Model file for the job. Use its own axes, mm. Face numbers are marked on the shaded views. A direction names the side the tool comes from. Round coordinates to 2 decimals unless told otherwise and drop trailing zeros. Order: outer loops, then holes, each group sorted by start corner. A loop starts at its lowest first (then second) coordinate and runs counter-clockwise, first axis right, second up. Notation, with made-up numbers: (53, 64.5) -> (59, 64.5) arc R24 cw to (59, 90.5) -> close; hole circle Ø11 at (43.25, 20). An arc over 180 degrees is marked (long way). Put each result on its own line as item: value. Start each with the question number.
Q1. Cut at A-A, the plane x = 178.5. List the corners of the cut face in (y, z).
Q2. Cut at C-C, the plane x = 63. List the corners of the cut face in (y, z).
Q3. Probe L1, parallel to Z at x = 64, y = 28.5; L2, parallel to X at y = 44.5, z = -21.5; L3, parallel to Z at x = 27.5, y = 46. List the from-to ranges inside material, lowest first.
Q4. 3-axis set-ups, long thin cutter, end or side, ignore diameter. For the marked faces 1, 2 and 3: which of +Z, -Z, +X, -X, +Y, -Y reach the whole face in a straight line?
Q5. Cut at B-B, the plane z = -132.5. List the corners of the cut face in (x, y), and give its area (3 significant figures).
Q6. Cut at D-D, the plane z = -160. List the corners of the cut face in (x, y), and give its area (3 significant figures).
Q7. Pull direction X, two halves, no side cores. Call the marked faces 4, 5, 6 and 7: released by +X, released by -X, zero draft, split by the parting line, or undercut.
Q8. Flat gauge pins, fed straight in: P1, Ø3, axis at y = 14, z = -142.5, coming from the +X side; P2, Ø2.5, axis at x = 47.5, y = 30, coming from the +Z side; P3, Ø6, axis at x = 162, z = -55, coming from the -Y side; P4, Ø6, axis at x = 156, z = -109, coming from the -Y side. Where does each tip first touch, or does it go through?
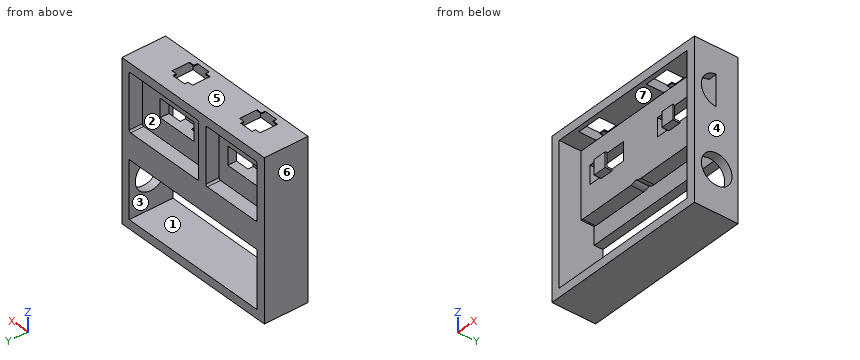
from build123d import *

# Parameters (mm, degrees)
SKETCH2_W            = 195
SKETCH2_H            = 180
BOSS_EXTRUDE1_DEPTH  = 50
CUT_EXTRUDE1_DEPTH   = 15
BOSS_EXTRUDE4_DEPTH  = 50
SKETCH14_W           = 70
SKETCH14_H           = 65
SKETCH14_W_2         = 95
BOSS_EXTRUDE8_DEPTH  = 35
SHELL2_OUTLINE_W     = 175
SHELL2_OUTLINE_H     = 65
SHELL2_DEPTH         = 75
SHELL2_2_OUTLINE_W   = 175
SHELL2_2_OUTLINE_H   = 95
SHELL2_2_DEPTH       = 25
SHELL2_START         = 25
SHELL2_3_DEPTH       = 15
SKETCH15_W           = 46
SKETCH15_H           = 21
CUT_EXTRUDE2_DEPTH   = 10
SKETCH16_W           = 46
SKETCH16_H           = 21
CUT_EXTRUDE3_DEPTH   = 10
SKETCH17_W           = 7.5
SKETCH17_H           = 8
BOSS_EXTRUDE10_DEPTH = 2
SKETCH18_W           = 15
SKETCH18_H           = 2
BOSS_EXTRUDE11_DEPTH = 15
CUT_EXTRUDE5_DEPTH   = 10
CUT_EXTRUDE6_DEPTH   = 9
SKETCH25_W           = 7.379331851
SKETCH25_H           = 8
SKETCH25_W_2         = 7.620668149
BOSS_EXTRUDE12_DEPTH = 2
SKETCH26_W           = 15
SKETCH26_H           = 2
BOSS_EXTRUDE13_DEPTH = 15
SKETCH27_R           = 17.5
CUT_EXTRUDE10_DEPTH  = 10
BOSS_EXTRUDE14_START = -10
BOSS_EXTRUDE14_DEPTH = 10


# Read off the part's stored shape, not the designer's step: Shell2
with BuildPart() as part:
    # Sketch2 → Boss-Extrude1 (new body)
    with BuildSketch(Plane(origin=(0, 0, 0), x_dir=(1, 0, 0), z_dir=(0, 1, 0))):
        with Locations((97.5, 90)):
            Rectangle(SKETCH2_W, SKETCH2_H)
    extrude(amount=BOSS_EXTRUDE1_DEPTH)

    # Sketch3 → Cut-Extrude1 (cut)
    with BuildSketch(Plane(origin=(0, 50, 0), x_dir=(1, 0, 0), z_dir=(0, 1, 0))):
        with BuildLine():
            Line((90, 12), (90, 73))
            ThreePointArc((90, 73), (90.585786438, 74.414213562), (92, 75))
            Line((92, 75), (183, 75))
            ThreePointArc((183, 75), (184.414213562, 74.414213562), (185, 73))
            Line((185, 73), (185, 12))
            ThreePointArc((185, 12), (184.414213562, 10.585786438), (183, 10))
            Line((183, 10), (92, 10))
            ThreePointArc((92, 10), (90.585786438, 10.585786438), (90, 12))
        make_face()
        with BuildLine():
            Line((12, 10), (78, 10))
            ThreePointArc((78, 10), (79.414213562, 10.585786438), (80, 12))
            Line((80, 12), (80, 73))
            ThreePointArc((80, 73), (79.414213562, 74.414213562), (78, 75))
            Line((78, 75), (12, 75))
            ThreePointArc((12, 75), (10.585786438, 74.414213562), (10, 73))
            Line((10, 73), (10, 12))
            ThreePointArc((10, 12), (10.585786438, 10.585786438), (12, 10))
        make_face()
    extrude(amount=-CUT_EXTRUDE1_DEPTH, mode=Mode.SUBTRACT)

    # Sketch6 → Boss-Extrude4 (add)
    with BuildSketch(Plane(origin=(0, 50, 0), x_dir=(1, 0, 0), z_dir=(0, 1, 0))):
        Polygon((0, 180), (185, 180), (195, 180), (195, 95), (185, 95), (0, 95), align=None)
        with BuildLine():
            Line((185, 168), (185, 107))
            ThreePointArc((185, 107), (184.414213562, 105.585786438), (183, 105))
            Line((183, 105), (92, 105))
            ThreePointArc((92, 105), (90.585786438, 105.585786438), (90, 107))
            Line((90, 107), (90, 168))
            ThreePointArc((90, 168), (90.585786438, 169.414213562), (92, 170))
            Line((92, 170), (183, 170))
            ThreePointArc((183, 170), (184.414213562, 169.414213562), (185, 168))
        make_face(mode=Mode.SUBTRACT)
        with BuildLine():
            Line((80, 107), (80, 168))
            ThreePointArc((80, 168), (79.414213562, 169.414213562), (78, 170))
            Line((78, 170), (12, 170))
            ThreePointArc((12, 170), (10.585786438, 169.414213562), (10, 168))
            Line((10, 168), (10, 107))
            ThreePointArc((10, 107), (10.585786438, 105.585786438), (12, 105))
            Line((12, 105), (78, 105))
            ThreePointArc((78, 105), (79.414213562, 105.585786438), (80, 107))
        make_face(mode=Mode.SUBTRACT)
    extrude(amount=BOSS_EXTRUDE4_DEPTH)

    # Sketch14 → Boss-Extrude8 (add)
    with BuildSketch(Plane(origin=(0, 50, 0), x_dir=(1, 0, 0), z_dir=(0, 1, 0))):
        with Locations((45, 137.5)):
            Rectangle(SKETCH14_W, SKETCH14_H)
        with Locations((137.5, 137.5)):
            Rectangle(SKETCH14_W_2, SKETCH14_H)
    extrude(amount=BOSS_EXTRUDE8_DEPTH)

    # Shell2 outline → Shell2 (cut)
    with BuildSketch(Plane(origin=(0, 0, 0), x_dir=(1, 0, 0), z_dir=(0, 1, 0))):
        with Locations((97.5, 137.5)):
            Rectangle(SHELL2_OUTLINE_W, SHELL2_OUTLINE_H)
    extrude(amount=SHELL2_DEPTH, mode=Mode.SUBTRACT)

    # Shell2 2 outline → Shell2 2 (cut)
    with BuildSketch(Plane(origin=(0, 0, 0), x_dir=(1, 0, 0), z_dir=(0, 1, 0))):
        with Locations((97.5, 57.5)):
            Rectangle(SHELL2_2_OUTLINE_W, SHELL2_2_OUTLINE_H)
    extrude(amount=SHELL2_2_DEPTH, mode=Mode.SUBTRACT)

    # Shell2 3 outline → Shell2 3 (cut)
    with BuildSketch(Plane(origin=(0, 0, 0), x_dir=(1, 0, 0), z_dir=(0, 1, 0)).offset(SHELL2_START)):
        with BuildLine():
            Line((10, 105), (10, 84.832159566))
            ThreePointArc((10, 84.832159566), (10.996484877, 84.957966273), (12, 85))
            Line((12, 85), (78, 85))
            ThreePointArc((78, 85), (81.676851089, 84.422817781), (85, 82.746794345))
            ThreePointArc((85, 82.746794345), (88.323148911, 84.422817781), (92, 85))
            Line((92, 85), (183, 85))
            ThreePointArc((183, 85), (184.003515123, 84.957966273), (185, 84.832159566))
            Line((185, 84.832159566), (185, 105))
            Line((185, 105), (10, 105))
        make_face()
    extrude(amount=SHELL2_3_DEPTH, mode=Mode.SUBTRACT)

    # SurfaceCut2
    split(bisect_by=Plane(origin=(0, 50, 0), x_dir=(1, 0, 0), z_dir=(0, 1, 0)), keep=Keep.BOTTOM)

    # Sketch15 → Cut-Extrude2 (cut)
    with BuildSketch(Plane(origin=(0, 35, 0), x_dir=(1, 0, 0), z_dir=(0, 1, 0))):
        with Locations((45, 42.5)):
            Rectangle(SKETCH15_W, SKETCH15_H)
    extrude(amount=-CUT_EXTRUDE2_DEPTH, mode=Mode.SUBTRACT)

    # Sketch16 → Cut-Extrude3 (cut)
    with BuildSketch(Plane(origin=(0, 35, 0), x_dir=(1, 0, 0), z_dir=(0, 1, 0))):
        with Locations((137.5, 42.5)):
            Rectangle(SKETCH16_W, SKETCH16_H)
    extrude(amount=-CUT_EXTRUDE3_DEPTH, mode=Mode.SUBTRACT)

    # Sketch17 → Boss-Extrude10 (add)
    with BuildSketch(Plane.XY.offset(-53)):
        with Locations((48.75, 21)):
            Rectangle(SKETCH17_W, SKETCH17_H)
        with Locations((41.25, 21)):
            Rectangle(SKETCH17_W, SKETCH17_H)
    extrude(amount=-BOSS_EXTRUDE10_DEPTH)

    # Sketch18 → Boss-Extrude11 (add)
    with BuildSketch(Plane.XY.offset(-53)):
        with Locations((45, 18)):
            Rectangle(SKETCH18_W, SKETCH18_H)
    extrude(amount=BOSS_EXTRUDE11_DEPTH)

    # Sketch20 → Cut-Extrude5 (cut)
    with BuildSketch(Plane.XY):
        Polygon((37, 29), (31, 29), (31, 9), (37, 9), (37, 5), (45, 5), (53, 5), (53, 9), (59, 9), (59, 19), (59, 29), (53, 29), (53, 33), (43.658923735, 33), (37, 33), align=None)
    cut_extrude5 = extrude(amount=-CUT_EXTRUDE5_DEPTH, mode=Mode.SUBTRACT)

    # Sketch21 → Cut-Extrude6 (cut)
    with BuildSketch(Plane(origin=(0, 0, -10), x_dir=(-1, 0, 0), z_dir=(0, 0, -1))):
        Polygon((-53, 5), (-31, 5), (-31, 12.573974865), (-31, 33), (-52.681459042, 33), (-59, 33), (-59, 15.767843478), (-59, 5), align=None)
    cut_extrude6 = extrude(amount=-CUT_EXTRUDE6_DEPTH, mode=Mode.SUBTRACT)

    # Sketch25 → Boss-Extrude12 (add)
    with BuildSketch(Plane.XY.offset(-53)):
        with Locations((133.810334075, 21)):
            Rectangle(SKETCH25_W, SKETCH25_H)
        with Locations((141.310334075, 21)):
            Rectangle(SKETCH25_W_2, SKETCH25_H)
    extrude(amount=-BOSS_EXTRUDE12_DEPTH)

    # Sketch26 → Boss-Extrude13 (add)
    with BuildSketch(Plane.XY.offset(-53)):
        with Locations((137.620668149, 18)):
            Rectangle(SKETCH26_W, SKETCH26_H)
    extrude(amount=BOSS_EXTRUDE13_DEPTH)

    # Mirror4: Cut-Extrude5, Cut-Extrude6 across plane
    add(cut_extrude5.mirror(Plane(origin=(91.25, 0, 0), x_dir=(0, 0, 1), z_dir=(1, 0, 0))), mode=Mode.SUBTRACT)
    add(cut_extrude6.mirror(Plane(origin=(91.25, 0, 0), x_dir=(0, 0, 1), z_dir=(1, 0, 0))), mode=Mode.SUBTRACT)

    # Sketch27 → Cut-Extrude10 (cut)
    with BuildSketch(Plane.ZY.offset(-185)):
        with Locations((-132.5, 25.5)):
            Circle(SKETCH27_R)
        with BuildLine():
            ThreePointArc((-64.985711369, 25), (-59.689166602, 12.950099602), (-47.492855685, 8))
            ThreePointArc((-47.492855685, 8), (-35.296544767, 12.950099602), (-30, 25))
            Line((-30, 25), (-64.985711369, 25))
        make_face()
        with BuildLine():
            Line((-64.985711369, 25), (-30, 25))
            ThreePointArc((-30, 25), (-29.994641855, 25.249974481), (-29.992855685, 25.5))
            ThreePointArc((-29.992855685, 25.5), (-47.742881204, 42.99821383), (-64.985711369, 25))
        make_face()
    extrude(amount=-CUT_EXTRUDE10_DEPTH, mode=Mode.SUBTRACT)

    # Sketch28 → Boss-Extrude14 (add)
    with BuildSketch(Plane(origin=(195, 0, 0), x_dir=(0, 0, -1), z_dir=(1, 0, 0)).offset(BOSS_EXTRUDE14_START)):
        with BuildLine():
            Line((30, 25), (64.985711369, 25))
            ThreePointArc((64.985711369, 25), (47.492855685, 43), (30, 25))
        make_face()
    extrude(amount=BOSS_EXTRUDE14_DEPTH)


solid = part.part
Ans:
1. outline: (0, -180) -> (50, -180) -> (50, -170) -> (0, -170) -> close; (0, -10) -> (25, -10) -> (25, -85) -> (40, -85) -> (40, -105) -> (50, -105) -> (50, -75) -> (35, -75) -> (35, -10) -> (50, -10) -> (50, 0) -> (0, 0) -> close
2. outline: (0, -180) -> (50, -180) -> (50, -170) -> (0, -170) -> close; (0, -10) -> (25, -10) -> (25, -32) -> (35, -32) -> (35, -10) -> (50, -10) -> (50, 0) -> (0, 0) -> close; (25, -85) -> (40, -85) -> (40, -105) -> (50, -105) -> (50, -75) -> (35, -75) -> (35, -53) -> (25, -53) -> close
3. L1: z = -180 to -170, -85 to -53, -32 to 0
3. L2: x = 0 to 10, 80 to 90, 185 to 195
3. L3: z = -180 to -170, -105 to -75, -10 to 0
4. face 1: +Y, -Y
4. face 2: +Y
4. face 3: -Y
5. outline: (0, 0) -> (10, 0) -> (10, 50) -> (0, 50) -> close; (185, 0) -> (195, 0) -> (195, 8) -> (185, 8) -> close; (185, 43) -> (195, 43) -> (195, 50) -> (185, 50) -> close
5. area: 650 mm^2
6. outline: (0, 0) -> (10, 0) -> (10, 50) -> (0, 50) -> close; (185, 0) -> (195, 0) -> (195, 50) -> (185, 50) -> close
6. area: 1,000 mm^2
7. face 4: released by +X
7. face 5: zero draft
7. face 6: released by -X
7. face 7: undercut
8. P1: stops at x = 10
8. P2: stops at z = -10
8. P3: stops at y = 25
8. P4: passes through
